from build123d import *

# Parameters (mm, degrees)
F1_W = 50.8
F1_H = 50.8


with BuildPart() as f2:
    # F2: sweep along a path in F0
    with BuildLine(Plane.XY) as f2_path:
        Line((-1219.2, 609.6), (-1219.2, -609.6))
        Line((-1219.2, -609.6), (1219.2, -609.6))
        Line((1219.2, -609.6), (1219.2, 609.6))
        Line((1219.2, 609.6), (-1219.2, 609.6))
    # F1 (on Front) → F2 (sweep)
    with BuildSketch(Plane.XZ):
        with Locations((-1219.2, 0)):
            Rectangle(F1_W, F1_H)
    sweep(path=f2_path.line, transition=Transition.RIGHT)


solid = f2.part
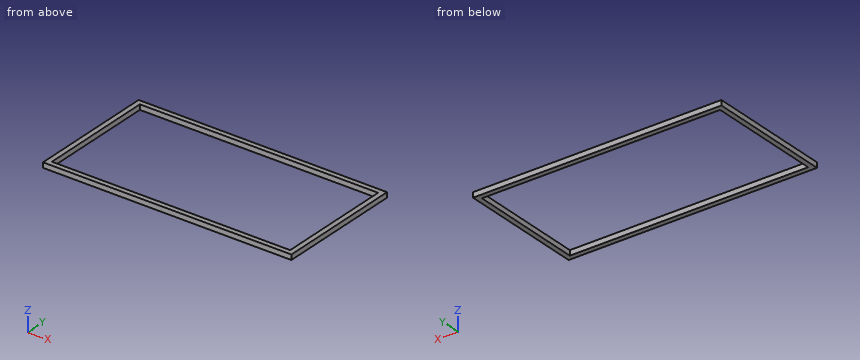
Work out the finished part from the listing and answer in its coordinate system (mm). Round coordinates to 2 decimals unless told otherwise and drop trailing zeros. Write each loop counter-clockwise with the first axis right and the second up, starting at its lowest first coordinate (ties: lowest second). Pieces come first, ordered by that corner, then holes.
1) A cutting plane is placed at C-C (y = 538). Give the vertices of the cut face in (x, z).
2) A cutting plane is placed at B-B (x = -197). Give the vertices of the cut face in (y, z).
3) Straight lines are drawn through the part: line 1 (X direction, y = 282, z = 23.5); line 2 (Y direction, x = -569.5, z = -23). For each, find the intervals that lie inside material, in ascending order.
4) A cutting plane is placed at A-A (z = 15). Give the vertices of the cut face in (x, y).
Completed:
1. outline: (-1244.6, -25.4) - (-1193.8, -25.4) - (-1193.8, 25.4) - (-1244.6, 25.4) - close; (1193.8, -25.4) - (1244.6, -25.4) - (1244.6, 25.4) - (1193.8, 25.4) - close
2. outline: (-635, -25.4) - (-584.2, -25.4) - (-584.2, 25.4) - (-635, 25.4) - close; (584.2, -25.4) - (635, -25.4) - (635, 25.4) - (584.2, 25.4) - close
3. line 1: x = -1244.6 to -1193.8, 1193.8 to 1244.6
3. line 2: y = -635 to -584.2, 584.2 to 635
4. outline: (-1244.6, -635) - (1244.6, -635) - (1244.6, 635) - (-1244.6, 635) - close; hole (-1193.8, -584.2) - (1193.8, -584.2) - (1193.8, 584.2) - (-1193.8, 584.2) - close
